Build history of the part. All positions in model axes, mm. Face numbers are marked on the shaded views. Coordinates: 2 decimals unless noted, no trailing zeros. Order: outer loops, then holes, each group sorted by start corner. A loop starts at its lowest first (then second) coordinate and runs counter-clockwise, first axis right, second up. Notation, with made-up numbers: (76, 44) - (114, 44) arc R16 ccw to (114, 69) - close; hole circle Ø3 at (82.5, 36.25). An arc over 180 degrees is marked (long way). One line per item, written item: value.
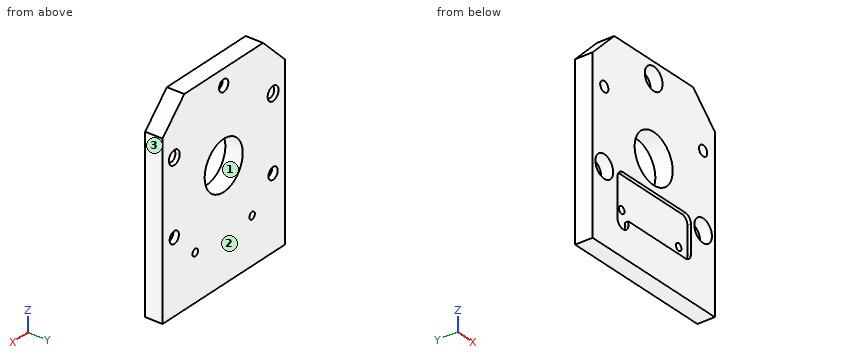
Autodesk Inventor part; units mm, degrees
ref_plane "YZ Plane" through (0, 0, 0) normal (1, 0, 0) x (0, 1, 0)
ref_plane "XZ Plane" through (0, 0, 0) normal (0, 1, 0) x (-1, 0, 0)
ref_plane "XY Plane" through (0, 0, 0) normal (0, 0, 1) x (1, 0, 0)
sketch "Sketch1" plane through (0, 0, 0) normal (0, 1, 0) x (-1, 0, 0)
  line L0 (-22.5, 28.5) -> (22.5, 28.5)
  line L1 (22.5, 28.5) -> (22.5, -28.5)
  line L2 (22.5, -28.5) -> (-22.5, -28.5)
  line L3 (-22.5, -28.5) -> (-22.5, 28.5)
  line L4 (-22.5, 28.5) -> (22.5, -28.5) construction
  line L5 (22.5, 28.5) -> (-22.5, -28.5) construction
  circle A0 centre (0, 0) radius 21 construction
  line L6 (0, -43.2) -> (0, 40.45)
  line L7 (22.5, -28.5) -> (-22.5, -28.5)
  line L8 (-22.5, -28.5) -> (-22.5, -31.25)
  line L9 (-22.5, -31.25) -> (22.5, -31.25)
  line L10 (22.5, -31.25) -> (22.5, -28.5)
  point P0 (0, 21)
  point P1 (-18.1865, -10.5)
  point P2 (18.1865, -10.5)
  dimension "d2" = 42
  dimension "d0" = 45
  dimension "d1" = 57
  dimension "d5" = 360
  dimension "d62" = 2.75
extrude "Extrusion1" add sketch "Sketch1" along normal blind 5
hole "Hole1" at (0, 0, 21) at (18.1865, 0, -10.5) at (-18.1865, 0, -10.5) direction (0, 1, 0) diameter 3.4 depth 8.8 tip angle 118 counterbore diameter 6.5 counterbore depth 3.4
sketch "Sketch2" plane through (0, 0, 0) normal (0, -1, 0) x (1, 0, 0)
  circle A0 centre (0, 0) radius 7
  dimension "d16" = 14
extrude "Extrusion2" cut sketch "Sketch2" against normal through all
sketch "Sketch3" plane through (0, 5, 0) normal (0, 1, 0) x (1, 0, 0)
  circle A0 centre (0, 0) radius 21 construction
  point P0 (18.1865, -10.5)
  point P1 (0, 21)
  point P2 (-18.1865, -10.5)
  dimension "d19" = 42
  dimension "d22" = 360
hole "Hole2" at (18.1865, 5, 10.5) at (-18.1865, 5, 10.5) direction (0, -1, 0) diameter 3 depth 8.8 tip angle 118
chamfer "Chamfer1" distance 0.5 angle 60 2 edges at (-18.1865, 5, 9) (18.1865, 5, 9) measured on face at (-0.2813, 5, -23.1497)
sketch "Sketch5" plane through (0, 0, 0) normal (0, -1, 0) x (1, 0, 0)
  line L0 (-13.3095, -20.83) -> (13.6905, -20.83)
  line L1 (13.6905, -20.83) -> (13.6905, -8.83)
  line L2 (13.6905, -8.83) -> (-13.3095, -8.83)
  line L3 (-13.3095, -8.83) -> (-13.3095, -20.83)
  line L4 (-13.3095, -20.83) -> (13.6905, -8.83) construction
  line L5 (13.6905, -20.83) -> (-13.3095, -8.83) construction
  line L6 (0, -36.4441) -> (0, 10.0043) construction
  circle A0 centre (0, 0) radius 7
  point P0 (0.1905, -14.83)
  point P1 (3.4689, -6.08)
  point P2 (-3.4689, -6.08)
  dimension "d34" = 12
  dimension "d35" = 27
  dimension "d36" = 13.3095
  dimension "d38" = 20.83
extrude "Extrusion3" cut sketch "Sketch5" against normal blind 1 contours L3 L2 L1 L0
sketch "Sketch6" plane through (0, 1, 0) normal (0, -1, 0) x (1, 0, 0)
  circle A0 centre (-10.4775, -18.036) radius 1.1414 construction
  line L0 (-13.3095, -20.83) -> (-13.3095, -8.83)
  line L1 (13.6905, -20.83) -> (-13.3095, -20.83)
  circle A1 centre (10.4775, -18.036) radius 1.164 construction
  line L2 (-10.4775, -18.036) -> (12.0154, -18.036) construction
  point P0 (0, 0)
  dimension "d41" = 2.832
  dimension "d42" = 2.794
  dimension "d43" = 20.955
hole "Hole3" at (10.4775, 1, -18.036) at (-10.4775, 1, -18.036) direction (0, 1, 0) diameter 2.013 depth 7.6 tip angle 118
sketch "Sketch7" plane through (0, 0, 0) normal (0, -1, 0) x (1, 0, 0)
  line L0 (13.6905, -20.83) -> (-13.3095, -20.83)
  circle A0 centre (-11.3095, -20.83) radius 2
  line L1 (-13.3095, -20.83) -> (-13.3095, -8.83)
  line L2 (-9.3095, -20.83) -> (-9.3095, -23.83)
  line L3 (-13.3095, -20.83) -> (-13.3095, -23.83)
  line L4 (-9.3095, -23.83) -> (-13.3095, -23.83)
  line L5 (22.5, -31.25) -> (-22.5, -31.25)
  point P0 (0, 0)
  point P1 (-9.3095, -18.08)
  point P2 (-13.3095, -20.83)
  dimension "d51" = 4
  dimension "d63" = 3
extrude "Extrusion4" cut sketch "Sketch7" against normal blind 1
sketch "Sketch8" plane through (-22.5, 0, 28.5) normal (0, 0, 1) x (1, 0, 0)
  line L0 (25.75, 3.4) -> (19.25, 3.4)
  line L1 (0, 0) -> (45, 0)
  line L2 (45, 0) -> (45, 5)
  line L3 (0, 5) -> (45, 5)
  line L4 (0, 0) -> (0, 5)
  point P0 (22.5, 0)
extrude "Extrusion5" cut sketch "Sketch8" against normal blind 3
fillet "Fillet1" radius 2 5 edges at (13.6905, 0.5, -20.83) (13.6905, 0.5, -8.83) (-13.3095, 0.5, -8.83) (-9.3095, 0.5, -23.83) (-13.3095, 0.5, -23.83)
sketch "Sketch11" plane through (0, 5, 0) normal (0, 1, 0) x (1, 0, 0)
  point P0 (0, 0)
chamfer "Chamfer3" distance 8 angle 45 2 edges at (22.5, 2.5, 25.5) (-22.5, 2.5, 25.5)
properties part number "encoder mount"
1. Band-saw the part on C-C, the plane x = 0. Give the cut face in (y, z).
Values found:
outline: (0, -31.25) - (5, -31.25) - (5, -7) - (0, -7) - (0, -8.83) - (1, -8.83) - (1, -20.83) - (0, -20.83) - close; (0, 7) - (5, 7) - (5, 19.3) - (3.4, 19.3) - (3.4, 17.75) - (0, 17.75) - close; (0, 24.25) - (3.4, 24.25) - (3.4, 22.7) - (5, 22.7) - (5, 25.5) - (0, 25.5) - close
2. Band-saw the part on D-D, the plane x = -6. Give the cut face in (y, z), and give its area (3 significant figures).
Values found:
outline: (0, -31.25) - (5, -31.25) - (5, -3.61) - (0, -3.61) - (0, -8.83) - (1, -8.83) - (1, -20.83) - (0, -20.83) - close; (0, 3.61) - (5, 3.61) - (5, 25.5) - (0, 25.5) - close
area: 236 mm2
3. Band-saw the part on A-A, the plane z = 10.5. Give the cut face in (x, y), and give its area (3 significant figures).
Values found:
outline: (-22.5, 0) - (-19.69, 0) - (-19.69, 4.13) - (-20.19, 5) - (-22.5, 5) - close; (-16.69, 0) - (16.69, 0) - (16.69, 4.13) - (16.19, 5) - (-16.19, 5) - (-16.69, 4.13) - close; (19.69, 0) - (22.5, 0) - (22.5, 5) - (20.19, 5) - (19.69, 4.13) - close
area: 194 mm2
4. Probe line 1 along Z through (x, y) = (0, 4.55); line 2 along X through (y, z) = (2.9, 10.5); line 3 along Z through (x, y) = (0, 0.85). List the from-to ranges inside material, lowest first.
Values found:
line 1: z = -31.25 to -7, 7 to 19.3, 22.7 to 25.5
line 2: x = -22.5 to -19.69, -16.69 to 16.69, 19.69 to 22.5
line 3: z = -31.25 to -20.83, -8.83 to -7, 7 to 17.75, 24.25 to 25.5
5. Flat gauge pins, fed straight in: P1, Ø2.5, axis at x = 18.19, z = -10.5, coming from the -Y side; P2, Ø4, axis at x = -18.19, z = -10.5, coming from the -Y side. Where does each tip first touch, or does it go through?
Values found:
P1: passes through
P2: stops at y = 3.4
6. Two-plate mould, pull along X, no slides. Class the marked faces 1, 2 and 3: pulls with the +X half, pulls with the -X half, needs draft (parallel to the pull), parting line crosses it, or undercut.
Values found:
face 1: undercut
face 2: needs draft
face 3: pulls with the +X half
7. Band-saw the part on B-B, the plane z = 21. Give the cut face in (x, y), and give its area (3 significant figures).
Values found:
outline: (-19, 0) - (-3.25, 0) - (-3.25, 3.4) - (-1.7, 3.4) - (-1.7, 5) - (-19, 5) - close; (1.7, 3.4) - (3.25, 3.4) - (3.25, 0) - (19, 0) - (19, 5) - (1.7, 5) - close
area: 162 mm2
